Model file for the job. Use its own axes, mm. Face numbers are marked on the shaded views. A direction names the side the tool comes from. Give positions to 0.01 mm unless a question says otherwise; leave off trailing zeros. Loops run counter-clockwise (first coordinate to the right, second up) from the corner with the lowest first, then second, coordinate; pieces in that order, holes last. Notation, with made-up numbers: (76, 49.25) - (127, 49.25) arc R22 cw to (127, 78.25) - close; hole circle Ø1 at (-17.5, 41). An arc over 180 degrees is marked (long way). Answer as CSV lines item,"result". Start each with the question number.
Item 1: Saw through at D-D on x = -13.25. Give the cut face in (y, z), plus the area to 3 significant figures.
Item 2: Saw through at A-A on z = -2. Give the cut face in (x, y).
Item 3: Saw through at B-B on y = 3. Give the cut face in (x, z).
Item 4: Pin check, flat tips, straight feed: pin 1 (6 mm diameter, centred on x = -5.5, y = 10.5, fed in from +Z); pin 2 (8.5 mm diameter, centred on y = 7, z = 1.5, fed in from -X). Stop position of each tip, or through.
Item 5: Tool access for the marked faces 5, 6 and 7: list every direction of +Z, -Z, +X, -X, +Y, -Y with a clear straight run to the whole face (end or side of a thin tool).
Item 6: Pull direction Y, two halves, no side cores. Call the marked faces 1, 2, 3 and 4: pulls with the +Y half, pulls with the -Y half, needs draft (parallel to the pull), parting line crosses it, or undercut.
Item 7: Drill centre lines: L1, parallel to Y at x = 0.75, z = 1.75; L2, parallel to Z at x = -14, y = 11.5; L3, parallel to X at y = 7.75, z = -3.25. Where is each one in solid material? Low to high. Write a range as from..to.
Item 8: Saw through at C-C on y = 7.5. Give the cut face in (x, z), plus the area to 3 significant figures.
from build123d import *

# Parameters (mm, degrees)
BOSS_EXTRUDE1_DEPTH = 19.88
SKETCH3_R           = 1.225
CUT_EXTRUDE1_DEPTH  = 3
CUT_EXTRUDE3_DEPTH  = 3


with BuildPart() as part:
    # Sketch1 → Boss-Extrude1 (new body)
    with BuildSketch(Plane(origin=(0, 0, 0), x_dir=(1, 0, 0), z_dir=(0, 1, 0))):
        with BuildLine():
            Line((-0.688375332, 9.340054497), (-0.688375332, -7.659945503))
            Line((-0.688375332, -7.659945503), (1.311624668, -7.659945503))
            Line((1.311624668, -7.659945503), (1.311624668, 11.340054497))
            ThreePointArc((1.311624668, 11.340054497), (1.018731449, 12.047161278), (0.311624668, 12.340054497))
            Line((0.311624668, 12.340054497), (-15.688375332, 12.340054497))
            Line((-15.688375332, 12.340054497), (-15.688375332, 10.340054497))
            Line((-15.688375332, 10.340054497), (-1.688375332, 10.340054497))
            ThreePointArc((-1.688375332, 10.340054497), (-0.981268551, 10.047161278), (-0.688375332, 9.340054497))
        make_face()
    extrude(amount=BOSS_EXTRUDE1_DEPTH)

    # Sketch3 → Cut-Extrude1 (cut, through all)
    with BuildSketch(Plane.XY.offset(-10.340054497)):
        with Locations((-8.688375332, 5.095)):
            Circle(SKETCH3_R)
        with Locations((-8.688375332, 14.785)):
            Circle(SKETCH3_R)
    extrude(amount=-CUT_EXTRUDE1_DEPTH, mode=Mode.SUBTRACT)

    # Sketch4 → Cut-Extrude3 (cut, through all)
    with BuildSketch(Plane.ZY.offset(0.688375332)):
        with BuildLine():
            Line((2.159945503, 17.915386938), (-3.840054497, 17.915386938))
            ThreePointArc((-3.840054497, 17.915386938), (-6.340054497, 15.415386938), (-3.840054497, 12.915386938))
            Line((-3.840054497, 12.915386938), (2.159945503, 12.915386938))
            ThreePointArc((2.159945503, 12.915386938), (4.659945503, 15.415386938), (2.159945503, 17.915386938))
        make_face()
        with BuildLine():
            Line((2.159945503, 6.964613062), (-3.840054497, 6.964613062))
            ThreePointArc((-3.840054497, 6.964613062), (-6.340054497, 4.464613062), (-3.840054497, 1.964613062))
            Line((-3.840054497, 1.964613062), (2.159945503, 1.964613062))
            ThreePointArc((2.159945503, 1.964613062), (4.659945503, 4.464613062), (2.159945503, 6.964613062))
        make_face()
    extrude(amount=-CUT_EXTRUDE3_DEPTH, mode=Mode.SUBTRACT)


solid = part.part
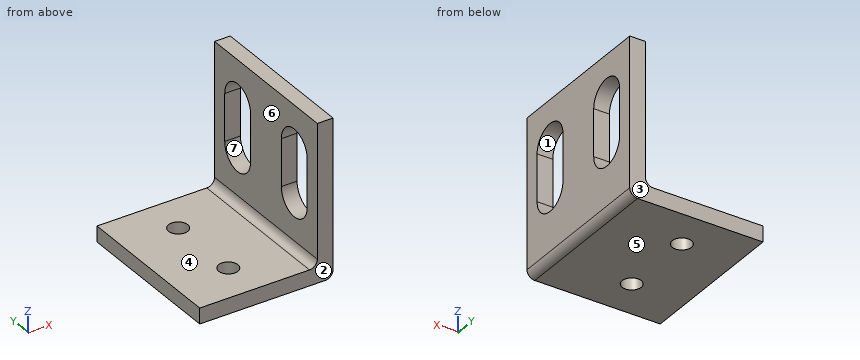
Responses:
1,outline,"(0, -12.34) - (19.88, -12.34) - (19.88, -10.34) - (0, -10.34) - close"
1,area,"39.8 mm2"
2,outline,"(-0.69, 0) - (1.31, 0) - (1.31, 1.96) - (-0.69, 1.96) - close; (-0.69, 6.96) - (1.31, 6.96) - (1.31, 12.92) - (-0.69, 12.92) - close; (-0.69, 17.92) - (1.31, 17.92) - (1.31, 19.88) - (-0.69, 19.88) - close"
3,outline,"(-15.69, -12.34) - (0.31, -12.34) arc R1 ccw to (1.31, -11.34) - (1.31, -5.87) - (-0.69, -5.87) - (-0.69, -9.34) arc R1 cw to (-1.69, -10.34) - (-15.69, -10.34) - close; (-0.69, 4.19) - (1.31, 4.19) - (1.31, 7.66) - (-0.69, 7.66) - close"
4,pin 1,"z = -10.34"
4,pin 2,"x = -0.69"
5,face 5,"-Z, +X, -X, +Y, -Y"
5,face 6,"+Z, -X, +Y, -Y"
5,face 7,"+X, -X"
6,face 1,"undercut"
6,face 2,"pulls with the -Y half"
6,face 3,"pulls with the +Y half"
6,face 4,"needs draft"
7,L1,"0..1.96, 6.96..12.92, 17.92..19.88"
7,L2,"-12.34..-10.34"
7,L3,"-0.69..1.31"
8,outline,"(-15.69, -12.34) - (0.31, -12.34) arc R1 ccw to (1.31, -11.34) - (1.31, 7.66) - (-0.69, 7.66) - (-0.69, -9.34) arc R1 cw to (-1.69, -10.34) - (-15.69, -10.34) - close"
8,area,"70.0 mm2"
